Verification items for the finished model (mm, model axes). Face numbers are marked on the shaded views. A direction names the side the tool comes from. Give positions to 0.01 mm unless a question says otherwise; leave off trailing zeros. Order: outer loops, then holes, each group sorted by start corner. A loop starts at its lowest first (then second) coordinate and runs counter-clockwise, first axis right, second up. Notation, with made-up numbers: (56.5, 74.5) - (63.5, 74.5) arc R19 cw to (63.5, 107.5) - close; hole circle Ø2 at (7.25, -13.5). An arc over 180 degrees is marked (long way). Answer as a JSON object with one key per item and string values.
```python
from build123d import *

# Parameters (mm, degrees)
CYLINDER_R           = 1
CYLINDER_DEPTH       = 26
CYLINDER_PITCH_ANGLE = 11
SKETCH001_W          = 1.861037
SKETCH001_H          = 10.545838
POCKET_DEPTH         = 3
SKETCH002_R          = 8.1
POCKET001_DEPTH      = 4.7
SKETCH003_R          = 7.5
POCKET002_DEPTH      = 5


with BuildPart() as cylinder:
    # Cylinder → Cylinder (new body)
    with BuildSketch(Plane.XY):
        Circle(CYLINDER_R)
    extrude(amount=CYLINDER_DEPTH)


with BuildPart() as cylinder_1:
    # Cylinder pitch: moved
    add(cylinder.part.rotate(Axis((0, 0, 0), (0, 1, 0)), CYLINDER_PITCH_ANGLE))


with BuildPart() as cylinder_2:
    # Cylinder placement: moved
    add(cylinder_1.part.moved(Location((-5, -11.5, -9.5))))


with BuildPart() as cut:
    # Sketch → Revolution (revolve)
    with BuildSketch(Plane.XY):
        Polygon((-6, 0), (-6, 11), (-5.489949, 11), (-4.5, 10.010051), (-3.510051, 11), (-3, 11), (-3, 15.62), (-2.489949, 15.62), (-1.5, 14.630051), (-0.510051, 15.62), (0, 15.62), (0, 0), align=None)
    revolve(axis=Axis((0, 0, 0), (1, 0, 0)))

    # Sketch001 → Pocket (cut)
    with BuildSketch(Plane(origin=(-6, 0, 0), x_dir=(0, -1, 0), z_dir=(-1, 0, 0))):
        with Locations((10.838202, -0.192388)):
            Rectangle(SKETCH001_W, SKETCH001_H)
    extrude(amount=-POCKET_DEPTH, mode=Mode.SUBTRACT)

    # Sketch002 → Pocket001 (cut)
    with BuildSketch(Plane(origin=(-6, 0, 0), x_dir=(0, -1, 0), z_dir=(-1, 0, 0))):
        Circle(SKETCH002_R)
    extrude(amount=-POCKET001_DEPTH, mode=Mode.SUBTRACT)

    # Sketch003 → Pocket002 (cut)
    with BuildSketch(Plane(origin=(-1.3, 0, 0), x_dir=(0, -1, 0), z_dir=(-1, 0, 0))):
        Circle(SKETCH003_R)
    extrude(amount=-POCKET002_DEPTH, mode=Mode.SUBTRACT)

    # Cut: cut Cylinder
    add(cylinder_2.part, mode=Mode.SUBTRACT)


solid = cut.part
```
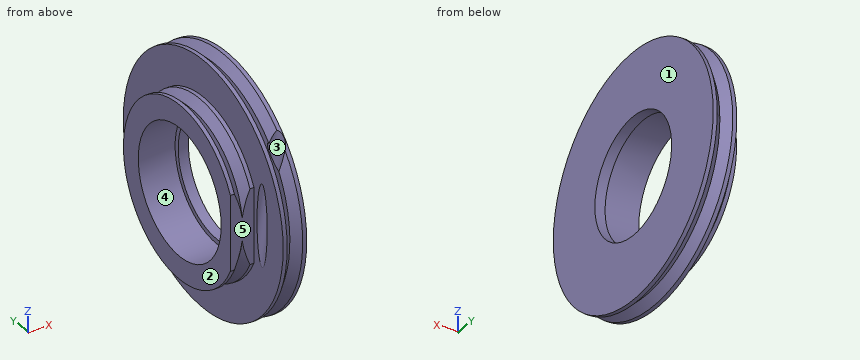
(1) Section check A-A (y = 0). Record the cut outline in (x, z), then the cut area to 3 significant figures.
Computed values:
{"outline": "(-6, -11) - (-5.49, -11) - (-4.5, -10.01) - (-3.51, -11) - (-3, -11) - (-3, -15.62) - (-2.49, -15.62) - (-1.5, -14.63) - (-0.51, -15.62) - (0, -15.62) - (0, -7.5) - (-1.3, -7.5) - (-1.3, -8.1) - (-6, -8.1) - close; (-6, 8.1) - (-1.3, 8.1) - (-1.3, 7.5) - (0, 7.5) - (0, 15.62) - (-0.51, 15.62) - (-1.5, 14.63) - (-2.49, 15.62) - (-3, 15.62) - (-3, 11) - (-3.51, 11) - (-4.5, 10.01) - (-5.49, 11) - (-6, 11) - close", "area": "60.2 mm²"}
(2) Release check for a two-part mould opening along X. For the marked faces 1, 2 and 3 record: pulls with the +X half, pulls with the -X half, needs draft (parallel to the pull), parting line crosses it, or undercut.
Computed values:
{"face 1": "pulls with the +X half", "face 2": "pulls with the -X half", "face 3": "undercut"}
(3) Access from +Z, -Z, +X, -X, +Y, -Y to the whole of each face (thin tool, end or side, straight path). Record for the marked faces 4 and 5.
Computed values:
{"face 4": "-X", "face 5": "+Z, -Z, -X, -Y"}
(4) Gauge pin test, flat ends, axial feed: pin 1 Ø2 at (x, y) = (-3.5, -3) entering from -Z; pin 2 Ø1.5 at (x, z) = (-5, -0.5) entering from -Y; pin 3 Ø1.5 at (x, y) = (-2, 7) entering from +Z. Record the tip position at first contact, or that the pin passes through.
Computed values:
{"pin 1": "stops at z = -15.47", "pin 2": "stops at y = -9.91", "pin 3": "stops at z = 14.23"}
(5) Material ranges on line 1 along Y through (x, z) = (-1.25, 5); line 2 along Z through (x, y) = (-2.95, 0); line 3 along Z through (x, y) = (-0.3, 0), recorded low to high. Write a range as [from, to].
Computed values:
{"line 1": "y = [-14.01, -11.9], [-11.1, -5.59], [5.59, 14.01]", "line 2": "z = [-15.62, -8.1], [8.1, 15.62]", "line 3": "z = [-15.62, -7.5], [7.5, 15.62]"}
(6) Section check C-C (x = -5). Record the cut outline in (y, z).
Computed values:
{"outline": "(-9.91, -3.51) arc R10.51 ccw (long way) to (-9.91, 3.51) - close; hole circle Ø16.2 at (0, 0)"}
(7) Section check B-B (z = 7). Count the separate pieces of the cut face and the enclosed holes in it, then the cut area to 3 significant figures.
Computed values:
{"separate pieces": "2", "enclosed holes": "1", "area": "81.4 mm²"}
